Read the model definition and answer for the solid it produces. Units are mm, in the model's axes. Give positions to 0.01 mm unless a question says otherwise; leave off trailing zeros. Order: outer loops, then holes, each group sorted by start corner. A loop starts at its lowest first (then second) coordinate and runs counter-clockwise, first axis right, second up. Notation, with made-up numbers: M 55.25,35 L 59.25,35 A31 cw 59.25,60 Z; hole C -22,-37.75 d7. An arc over 180 degrees is marked long. One line per item, written item: value.
from build123d import *

# Parameters (mm, degrees)
SKETCH008_R    = 8
HOLE005_DEPTH  = 25
SKETCH009_R    = 4
HOLE006_DEPTH  = 10
HOLE006_TIPS_R = 4


with BuildPart() as part:
    # Sketch007 → Revolution001 (revolve)
    with BuildSketch(Plane.XZ):
        with BuildLine():
            Line((0, 9), (-259, 9))
            ThreePointArc((-259, 9), (-263, 0), (-259, -9))
            Line((0, -9), (-259, -9))
            Line((0, 9), (0, -9))
        make_face()
    revolve(axis=Axis((0, 0, 0), (0, 0, 1)))

    # Sketch008 (on Face1 of Revolution001) → Hole005 (cut)
    with BuildSketch(Plane(origin=(0, 0, 9), x_dir=(-1, 0, 0), z_dir=(0, 0, 1))):
        Circle(SKETCH008_R)
    extrude(amount=-HOLE005_DEPTH, mode=Mode.SUBTRACT)

    # Sketch009 (on Face1 of Hole005) → Hole006 (cut)
    with BuildSketch(Plane(origin=(0, 0, 9), x_dir=(-1, 0, 0), z_dir=(0, 0, 1))):
        with Locations((-35, 35)):
            Circle(SKETCH009_R)
        with Locations((35, 35)):
            Circle(SKETCH009_R)
        with Locations((-35, -35)):
            Circle(SKETCH009_R)
        with Locations((35, -35)):
            Circle(SKETCH009_R)
    extrude(amount=-HOLE006_DEPTH, mode=Mode.SUBTRACT)

    # Hole006 tips → Hole006 tip 1 section 0
    with BuildSketch(Plane(origin=(0, 0, -1), x_dir=(-1, 0, 0), z_dir=(0, 0, 1)), mode=Mode.PRIVATE) as hole006_tip_1_s0:
        with Locations((-35, 35)):
            Circle(HOLE006_TIPS_R)
    loft([hole006_tip_1_s0.sketch, Vertex(35, -35, -3.403442)], mode=Mode.SUBTRACT)

    # Hole006 tips → Hole006 tip 2 section 0
    with BuildSketch(Plane(origin=(0, 0, -1), x_dir=(-1, 0, 0), z_dir=(0, 0, 1)), mode=Mode.PRIVATE) as hole006_tip_2_s0:
        with Locations((35, 35)):
            Circle(HOLE006_TIPS_R)
    loft([hole006_tip_2_s0.sketch, Vertex(-35, -35, -3.403442)], mode=Mode.SUBTRACT)

    # Hole006 tips → Hole006 tip 3 section 0
    with BuildSketch(Plane(origin=(0, 0, -1), x_dir=(-1, 0, 0), z_dir=(0, 0, 1)), mode=Mode.PRIVATE) as hole006_tip_3_s0:
        with Locations((-35, -35)):
            Circle(HOLE006_TIPS_R)
    loft([hole006_tip_3_s0.sketch, Vertex(35, 35, -3.403442)], mode=Mode.SUBTRACT)

    # Hole006 tips → Hole006 tip 4 section 0
    with BuildSketch(Plane(origin=(0, 0, -1), x_dir=(-1, 0, 0), z_dir=(0, 0, 1)), mode=Mode.PRIVATE) as hole006_tip_4_s0:
        with Locations((35, -35)):
            Circle(HOLE006_TIPS_R)
    loft([hole006_tip_4_s0.sketch, Vertex(-35, 35, -3.403442)], mode=Mode.SUBTRACT)


solid = part.part
1) Each of these flat-tipped pins is pushed along its axis until it touches: pin 1 Ø7 at (x, y) = (35, 35) entering from +Z; pin 2 Ø8 at (x, z) = (173, -6) entering from +Y; pin 3 Ø2 at (x, z) = (-15.5, -2.5) entering from +Y. Where does it stop, or does it pass through?
Reported:
pin 1: stops at z = -1.3
pin 2: stops at y = 200.18
pin 3: stops at y = 262.46
2) Find section C-C, the plane z = 4. Write down the section's boundary in (x, y).
Reported:
outline: C 0,0 d524.64; hole C -35,-35 d8; hole C -35,35 d8; hole C 0,0 d16; hole C 35,-35 d8; hole C 35,35 d8
3) Consider probe 1 along X at (y, z) = (35, 6); probe 2 along Y at (x, z) = (35, 3.5); probe 3 along Y at (x, z) = (35, 5.5). Determine where each line is inside the solid, lowest interval first.
Reported:
probe 1: x = -259.06 to -39, -31 to 31, 39 to 259.06
probe 2: y = -260.14 to -39, -31 to 31, 39 to 260.14
probe 3: y = -259.33 to -39, -31 to 31, 39 to 259.33
4) Determine the mould class of faces 1 (the face through (-4, 54, 9)), 2 (the face through (1.73, 7.81, 0.13)) for opening direction Y: +Y half, -Y half, draft (parallel to the pull), parting line (faces both ways), or undercut.
Reported:
face 1: draft
face 2: undercut
5) Find section A-A, the plane y = 0. Write down the section's boundary in (x, z) (3 decimals).
Reported:
outline: M -259,-9 L -8,-9 L -8,9 L -259,9 A12.125 ccw Z; M 8,-9 L 259,-9 A12.125 ccw 259,9 L 8,9 Z
